```python
from build123d import *

# Parameters (mm, degrees)
SKETCH2_R                 = 2.5
BOSS_EXTRUDE1_DEPTH       = 3
BOSS_EXTRUDE1_2_DEPTH     = 3
BOSS_EXTRUDE1_3_DEPTH     = 3
BOSS_EXTRUDE1_4_DEPTH     = 3
BOSS_EXTRUDE1_5_DEPTH     = 3
BOSS_EXTRUDE1_6_DEPTH     = 3
SKETCH4_W                 = 225
SKETCH4_H                 = 120
BOSS_EXTRUDE2_DEPTH       = 0.8
F_3_0MM_DOWEL_HOLE1_D     = 3
F_3_0MM_DOWEL_HOLE1_DEPTH = 4
CUT_EXTRUDE1_REACH        = 2.8
CHAMFER1_SIZE             = 66
CUT_EXTRUDE2_REACH        = 2.8
CHAMFER3_SIZE             = 70
CHAMFER3_SIZE2            = 23.885549322


with BuildPart() as part:
    # Sketch2 → Boss-Extrude1 (new body)
    with BuildSketch(Plane(origin=(0, 0, 0), x_dir=(1, 0, 0), z_dir=(0, 1, 0))):
        with Locations((101, 101)):
            Circle(SKETCH2_R)
    extrude(amount=BOSS_EXTRUDE1_DEPTH)



with BuildPart() as body_2:
    # Sketch2 → Boss-Extrude1 2 (new body)
    with BuildSketch(Plane(origin=(0, 0, 0), x_dir=(1, 0, 0), z_dir=(0, 1, 0))):
        with Locations((206, 68)):
            Circle(SKETCH2_R)
    extrude(amount=BOSS_EXTRUDE1_2_DEPTH)


with BuildPart() as body_3:
    # Sketch2 → Boss-Extrude1 3 (new body)
    with BuildSketch(Plane(origin=(0, 0, 0), x_dir=(1, 0, 0), z_dir=(0, 1, 0))):
        with Locations((214, 44)):
            Circle(SKETCH2_R)
    extrude(amount=BOSS_EXTRUDE1_3_DEPTH)


with BuildPart() as body_4:
    # Sketch2 → Boss-Extrude1 4 (new body)
    with BuildSketch(Plane(origin=(0, 0, 0), x_dir=(1, 0, 0), z_dir=(0, 1, 0))):
        with Locations((221, 25)):
            Circle(SKETCH2_R)
    extrude(amount=BOSS_EXTRUDE1_4_DEPTH)


with BuildPart() as body_5:
    # Sketch2 → Boss-Extrude1 5 (new body)
    with BuildSketch(Plane(origin=(0, 0, 0), x_dir=(1, 0, 0), z_dir=(0, 1, 0))):
        with Locations((41.5, 38)):
            Circle(SKETCH2_R)
    extrude(amount=BOSS_EXTRUDE1_5_DEPTH)


with BuildPart() as body_6:
    # Sketch2 → Boss-Extrude1 6 (new body)
    with BuildSketch(Plane(origin=(0, 0, 0), x_dir=(1, 0, 0), z_dir=(0, 1, 0))):
        with Locations((59, 96)):
            Circle(SKETCH2_R)
    extrude(amount=BOSS_EXTRUDE1_6_DEPTH)


with BuildPart() as part_1:
    add(part.part)

    add(body_2.part)  # Boss-Extrude2 merges body 2

    add(body_3.part)  # Boss-Extrude2 merges body 3

    add(body_4.part)  # Boss-Extrude2 merges body 4

    add(body_5.part)  # Boss-Extrude2 merges body 5

    add(body_6.part)  # Boss-Extrude2 merges body 6
    # Sketch4 → Boss-Extrude2 (add)
    with BuildSketch(Plane(origin=(0, 0, 0), x_dir=(1, 0, 0), z_dir=(0, 1, 0))):
        with Locations((112.5, 60)):
            Rectangle(SKETCH4_W, SKETCH4_H)
    extrude(amount=-BOSS_EXTRUDE2_DEPTH)

    # Ø3.0mm Dowel Hole1
    with Locations(Plane(origin=(0, 3, 0), x_dir=(1, 0, 0), z_dir=(0, 1, 0))):
        with Locations((59, 96), (101, 101), (206, 68), (214, 44), (221, 25), (41.5, 38)):
            Hole(F_3_0MM_DOWEL_HOLE1_D / 2, depth=F_3_0MM_DOWEL_HOLE1_DEPTH)

    # Sketch27 → Cut-Extrude1 (cut, up to next)
    with BuildSketch(Plane(origin=(0, 0, 0), x_dir=(1, 0, 0), z_dir=(0, 1, 0)), mode=Mode.PRIVATE) as cut_extrude1_sk1:
        Polygon((186, 8), (189, 8), (189, 12), (195, 12), (195, 8), (198, 8), (198, 4), (186, 4), align=None)
    cut_extrude1_tool1 = extrude(cut_extrude1_sk1.sketch, amount=-CUT_EXTRUDE1_REACH, mode=Mode.PRIVATE) & part_1.part
    add(cut_extrude1_tool1.solids().sort_by_distance((192, 0, -7.333333))[0], mode=Mode.SUBTRACT)
    # Sketch27 → Cut-Extrude1 (cut, up to next)
    with BuildSketch(Plane(origin=(0, 0, 0), x_dir=(1, 0, 0), z_dir=(0, 1, 0)), mode=Mode.PRIVATE) as cut_extrude1_sk2:
        Polygon((4, 6), (8, 6), (8, 9), (12, 9), (12, 15), (8, 15), (8, 18), (4, 18), align=None)
    cut_extrude1_tool2 = extrude(cut_extrude1_sk2.sketch, amount=-CUT_EXTRUDE1_REACH, mode=Mode.PRIVATE) & part_1.part
    add(cut_extrude1_tool2.solids().sort_by_distance((7.333333, 0, -12))[0], mode=Mode.SUBTRACT)

    # Chamfer1
    chamfer1_edges = [part_1.edges().sort_by_distance(p)[0] for p in [
        (0, -0.4, -120),
        (225, -0.4, -120),
    ]]
    chamfer(chamfer1_edges, length=CHAMFER1_SIZE)

    # Sketch28 → Cut-Extrude2 (cut, up to next)
    with BuildSketch(Plane(origin=(0, 0, 0), x_dir=(1, 0, 0), z_dir=(0, 1, 0)), mode=Mode.PRIVATE) as cut_extrude2_sk1:
        Polygon((52.388319297, 6.891877983), (52.388319297, 83.093591857), (124.427979621, 100.514856146), align=None)
    cut_extrude2_tool1 = extrude(cut_extrude2_sk1.sketch, amount=-CUT_EXTRUDE2_REACH, mode=Mode.PRIVATE) & part_1.part
    add(cut_extrude2_tool1.solids().sort_by_distance((76.401539, 0, -63.500109))[0], mode=Mode.SUBTRACT)
    # Sketch28 → Cut-Extrude2 (cut, up to next)
    with BuildSketch(Plane(origin=(0, 0, 0), x_dir=(1, 0, 0), z_dir=(0, 1, 0)), mode=Mode.PRIVATE) as cut_extrude2_sk2:
        Polygon((144.286671327, 114.724380441), (61.313270979, 6.891877983), (121.338711512, 6.891877983), align=None)
    cut_extrude2_tool2 = extrude(cut_extrude2_sk2.sketch, amount=-CUT_EXTRUDE2_REACH, mode=Mode.PRIVATE) & part_1.part
    add(cut_extrude2_tool2.solids().sort_by_distance((108.979551, 0, -42.836045))[0], mode=Mode.SUBTRACT)
    # Sketch28 → Cut-Extrude2 (cut, up to next)
    with BuildSketch(Plane(origin=(0, 0, 0), x_dir=(1, 0, 0), z_dir=(0, 1, 0)), mode=Mode.PRIVATE) as cut_extrude2_sk3:
        Polygon((152.485832321, 114.724380441), (129.537872506, 6.891877983), (176.515283586, 6.891877983), align=None)
    cut_extrude2_tool3 = extrude(cut_extrude2_sk3.sketch, amount=-CUT_EXTRUDE2_REACH, mode=Mode.PRIVATE) & part_1.part
    add(cut_extrude2_tool3.solids().sort_by_distance((152.846329, 0, -42.836045))[0], mode=Mode.SUBTRACT)
    # Sketch28 → Cut-Extrude2 (cut, up to next)
    with BuildSketch(Plane(origin=(0, 0, 0), x_dir=(1, 0, 0), z_dir=(0, 1, 0)), mode=Mode.PRIVATE) as cut_extrude2_sk4:
        Polygon((164.500557953, 105.19569086), (196.171947419, 73.524301395), (184.457582932, 18.478482617), align=None)
    cut_extrude2_tool4 = extrude(cut_extrude2_sk4.sketch, amount=-CUT_EXTRUDE2_REACH, mode=Mode.PRIVATE) & part_1.part
    add(cut_extrude2_tool4.solids().sort_by_distance((181.710029, 0, -65.732825))[0], mode=Mode.SUBTRACT)
    # Sketch28 → Cut-Extrude2 (cut, up to next)
    with BuildSketch(Plane(origin=(0, 0, 0), x_dir=(1, 0, 0), z_dir=(0, 1, 0)), mode=Mode.PRIVATE) as cut_extrude2_sk5:
        Polygon((198.888278472, 53.703367065), (211.405882256, 18.478482617), (193.110922879, 18.478482617), align=None)
    cut_extrude2_tool5 = extrude(cut_extrude2_sk5.sketch, amount=-CUT_EXTRUDE2_REACH, mode=Mode.PRIVATE) & part_1.part
    add(cut_extrude2_tool5.solids().sort_by_distance((201.135028, 0, -30.220111))[0], mode=Mode.SUBTRACT)
    # Sketch28 → Cut-Extrude2 (cut, up to next)
    with BuildSketch(Plane(origin=(0, 0, 0), x_dir=(1, 0, 0), z_dir=(0, 1, 0)), mode=Mode.PRIVATE) as cut_extrude2_sk6:
        Polygon((44.242680865, 83.093591857), (44.242680865, 52.616095827), (6.082421341, 25.506148765), align=None)
    cut_extrude2_tool6 = extrude(cut_extrude2_sk6.sketch, amount=-CUT_EXTRUDE2_REACH, mode=Mode.PRIVATE) & part_1.part
    add(cut_extrude2_tool6.solids().sort_by_distance((31.522594, 0, -53.738612))[0], mode=Mode.SUBTRACT)
    # Sketch28 → Cut-Extrude2 (cut, up to next)
    with BuildSketch(Plane(origin=(0, 0, 0), x_dir=(1, 0, 0), z_dir=(0, 1, 0)), mode=Mode.PRIVATE) as cut_extrude2_sk7:
        Polygon((13.630560586, 24.81954669), (34.944244067, 39.030171699), (47.359604213, 20.409100754), align=None)
    cut_extrude2_tool7 = extrude(cut_extrude2_sk7.sketch, amount=-CUT_EXTRUDE2_REACH, mode=Mode.PRIVATE) & part_1.part
    add(cut_extrude2_tool7.solids().sort_by_distance((31.978136, 0, -28.086273))[0], mode=Mode.SUBTRACT)
    # Sketch28 → Cut-Extrude2 (cut, up to next)
    with BuildSketch(Plane(origin=(0, 0, 0), x_dir=(1, 0, 0), z_dir=(0, 1, 0)), mode=Mode.PRIVATE) as cut_extrude2_sk8:
        Polygon((17.858383702, 18.478482617), (17.858383702, 6.891877983), (46.339021234, 6.891877983), align=None)
    cut_extrude2_tool8 = extrude(cut_extrude2_sk8.sketch, amount=-CUT_EXTRUDE2_REACH, mode=Mode.PRIVATE) & part_1.part
    add(cut_extrude2_tool8.solids().sort_by_distance((27.35193, 0, -10.75408))[0], mode=Mode.SUBTRACT)
    # Sketch28 → Cut-Extrude2 (cut, up to next)
    with BuildSketch(Plane(origin=(0, 0, 0), x_dir=(1, 0, 0), z_dir=(0, 1, 0)), mode=Mode.PRIVATE) as cut_extrude2_sk9:
        Polygon((66.741601703, 114.724380441), (69.339310273, 91.487471585), (93.043400976, 97.007602296), align=None)
    cut_extrude2_tool9 = extrude(cut_extrude2_sk9.sketch, amount=-CUT_EXTRUDE2_REACH, mode=Mode.PRIVATE) & part_1.part
    add(cut_extrude2_tool9.solids().sort_by_distance((76.374771, 0, -101.073151))[0], mode=Mode.SUBTRACT)
    # Sketch28 → Cut-Extrude2 (cut, up to next)
    with BuildSketch(Plane(origin=(0, 0, 0), x_dir=(1, 0, 0), z_dir=(0, 1, 0)), mode=Mode.PRIVATE) as cut_extrude2_sk10:
        Polygon((74.134214928, 115.550818021), (93.043400976, 102.813672146), (101.623087305, 115.550818021), align=None)
    cut_extrude2_tool10 = extrude(cut_extrude2_sk10.sketch, amount=-CUT_EXTRUDE2_REACH, mode=Mode.PRIVATE) & part_1.part
    add(cut_extrude2_tool10.solids().sort_by_distance((89.600234, 0, -111.305103))[0], mode=Mode.SUBTRACT)
    # Sketch28 → Cut-Extrude2 (cut, up to next)
    with BuildSketch(Plane(origin=(0, 0, 0), x_dir=(1, 0, 0), z_dir=(0, 1, 0)), mode=Mode.PRIVATE) as cut_extrude2_sk11:
        Polygon((136.446781668, 115.550818021), (126.813612387, 104.367776578), (109.710747348, 115.88819244), align=None)
    cut_extrude2_tool11 = extrude(cut_extrude2_sk11.sketch, amount=-CUT_EXTRUDE2_REACH, mode=Mode.PRIVATE) & part_1.part
    add(cut_extrude2_tool11.solids().sort_by_distance((124.323714, 0, -111.935596))[0], mode=Mode.SUBTRACT)
    # Sketch28 → Cut-Extrude2 (cut, up to next)
    with BuildSketch(Plane(origin=(0, 0, 0), x_dir=(1, 0, 0), z_dir=(0, 1, 0)), mode=Mode.PRIVATE) as cut_extrude2_sk12:
        Polygon((107.114322397, 112.702091574), (120.319340962, 103.610111579), (109.710747348, 101.653186543), align=None)
    cut_extrude2_tool12 = extrude(cut_extrude2_sk12.sketch, amount=-CUT_EXTRUDE2_REACH, mode=Mode.PRIVATE) & part_1.part
    add(cut_extrude2_tool12.solids().sort_by_distance((112.38147, 0, -105.988463))[0], mode=Mode.SUBTRACT)
    # Sketch28 → Cut-Extrude2 (cut, up to next)
    with BuildSketch(Plane(origin=(0, 0, 0), x_dir=(1, 0, 0), z_dir=(0, 1, 0)), mode=Mode.PRIVATE) as cut_extrude2_sk13:
        Polygon((203.456645773, 14.141546381), (220.018577109, 14.141546381), (220.018577109, 5.336468962), align=None)
    cut_extrude2_tool13 = extrude(cut_extrude2_sk13.sketch, amount=-CUT_EXTRUDE2_REACH, mode=Mode.PRIVATE) & part_1.part
    add(cut_extrude2_tool13.solids().sort_by_distance((214.497933, 0, -11.206521))[0], mode=Mode.SUBTRACT)

    # Chamfer3
    chamfer3_edges = [part_1.edges().sort_by_distance(p)[0] for p in [
        (0, -0.4, -54),
    ]]
    chamfer3_side = [part_1.faces().sort_by_distance(p)[0] for p in [
        (33, -0.4, -87),
    ]]
    chamfer(chamfer3_edges, length=CHAMFER3_SIZE, length2=CHAMFER3_SIZE2, reference=chamfer3_side[0])


solid = part_1.part
```
Geometry check sheet. Reference: the model listing, model coordinates, mm. A direction names the side the tool comes from. Coordinates: 2 decimals unless noted, no trailing zeros. Order: outer loops, then holes, each group sorted by start corner. A loop starts at its lowest first (then second) coordinate and runs counter-clockwise, first axis right, second up. Notation, with made-up numbers: (68.5, 43.25) - (75.5, 43.25) arc R15 ccw to (75.5, 66.25) - close; hole circle Ø3 at (87.5, -9). An arc over 180 degrees is marked (long way). Answer in a Markdown table with one row per item. Add a question column.
1. Material ranges on L1, parallel to X at y = 1.45, z = -44; L2, parallel to X at y = 1.3, z = -38; L3, parallel to Z at x = 41.5, y = 1.5, recorded low to high. Write a range as [from, to].
2. Section check B-B (x = 180.5). Enter the section's corners in (y, z).
3. Gauge pin test, flat ends, axial feed: pin 1 Ø0.9 at (y, z) = (-0.5, -68) entering from -X; pin 2 Ø0.6 at (x, y) = (206, 0) entering from -Z; pin 3 Ø1.5 at (y, z) = (0, -99.5) entering from +X. Record the tip position at first contact, or that the pin passes through.
4. Access from +Z, -Z, +X, -X, +Y, -Y to the whole of each face (thin tool, end or side, straight path). Record for faces 4 (the face through (131.7, -0.39, -110.04)), 5 (the face through (100.67, 1.48, -103.48)), 6 (the face through (59, 3, -94)).
5. Section check A-A (y = 1.6). Give the number of separate pieces and of enclosed holes in the cut face, plus the area to 3 significant figures.
6. Draft check along Z on faces 1 (the face through (208.31, 1.48, -67.04)), 2 (the face through (180.115, -0.394, -89.582)), 3 (the face through (129, 0, -38)). Enter one of: +Z half, -Z half, draft (parallel to the pull), parting line (faces both ways), or undercut.
Data:
| question | item | result |
|---|---|---|
| 1 | L1 | x = [211.5, 212.5], [215.5, 216.5] |
| 1 | L2 | x = [39, 40], [43, 44] |
| 1 | L3 | z = [-40.5, -39.5], [-36.5, -35.5] |
| 2 | outline | (-0.8, -98.5) - (0, -98.5) - (0, -89.2) - (-0.8, -89.2) - close; (-0.8, -35.67) - (0, -35.67) - (0, 0) - (-0.8, 0) - close |
| 3 | pin 1 | stops at x = 25.25 |
| 3 | pin 2 | stops at z = -73.3 |
| 3 | pin 3 | stops at x = 180.25 |
| 4 | face 4 | +Y, -Y |
| 4 | face 5 | +Y |
| 4 | face 6 | +Z, -Z, +X, -X, +Y |
| 5 | separate pieces | 6 |
| 5 | enclosed holes | 6 |
| 5 | area | 75.4 mm² |
| 6 | face 1 | parting line |
| 6 | face 2 | undercut |
| 6 | face 3 | draft |
